Input: part model. Units: mm. Frame: model coordinates. Face numbers are marked on the shaded views. A direction names the side the tool comes from. Round coordinates to 2 decimals unless told otherwise and drop trailing zeros. Order: outer loops, then holes, each group sorted by start corner. A loop starts at its lowest first (then second) coordinate and runs counter-clockwise, first axis right, second up. Notation, with made-up numbers: (-25, 35.25) -> (5, 35.25) arc R5 ccw to (5, 41.25) -> close; hole circle Ø11 at (2.25, 29.5). An arc over 180 degrees is marked (long way). Use a Markdown table: item, result.
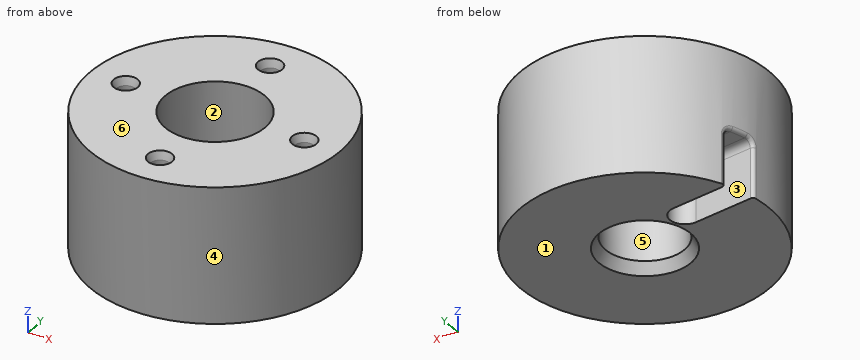
from build123d import *

# Parameters (mm, degrees)
SKETCH_1_R          = 17.5
EXTRUDE_1_DEPTH     = 19
SKETCH_2_R          = 1.3
CUT_EXTRUDE_1_DEPTH = 8
SKETCH_4_R          = 7
CUT_EXTRUDE_3_DEPTH = 9
SKETCH_5_R          = 5.55
CUT_EXTRUDE_4_DEPTH = 10
CUT_EXTRUDE_START   = -8
CUT_EXTRUDE_6_DEPTH = 8
FILLET_1_R          = 1
FILLET_2_R          = 0.5
CHAMFER_1_SIZE      = 0.9
CHAMFER_1_SIZE2     = 1.558845727
CHAMFER_2_SIZE      = 0.4
CHAMFER_2_SIZE2     = 1.098990968


with BuildPart() as part:
    # 草图1 → 凸台-拉伸1 (new body)
    with BuildSketch(Plane.XY):
        Circle(SKETCH_1_R)
    extrude(amount=-EXTRUDE_1_DEPTH)

    # 草图2 → 切除-拉伸1 (cut)
    with BuildSketch(Plane.XY):
        with Locations((12.5, 0)):
            Circle(SKETCH_2_R)
        with Locations((0, -12.5)):
            Circle(SKETCH_2_R)
        with Locations((-12.5, 0)):
            Circle(SKETCH_2_R)
        with Locations((0, 12.5)):
            Circle(SKETCH_2_R)
    extrude(amount=-CUT_EXTRUDE_1_DEPTH, mode=Mode.SUBTRACT)

    # 草图4 → 切除-拉伸3 (cut)
    with BuildSketch(Plane.XY):
        Circle(SKETCH_4_R)
    extrude(amount=-CUT_EXTRUDE_3_DEPTH, mode=Mode.SUBTRACT)

    # 草图5 → 切除-拉伸4 (cut)
    with BuildSketch(Plane.XY.offset(-9)):
        Circle(SKETCH_5_R)
    extrude(amount=-CUT_EXTRUDE_4_DEPTH, mode=Mode.SUBTRACT)

    # 草图11 → 切除-拉伸6 (cut)
    with BuildSketch(Plane(origin=(0, 0, -19), x_dir=(-1, 0, 0), z_dir=(0, 0, -1)).offset(CUT_EXTRUDE_START)):
        with BuildLine():
            ThreePointArc((17.194499347, 3.255640061), (16.671203225, 5.32174624), (15.900621658, 7.308914482))
            Line((15.900621658, 7.308914482), (7.74531425, 6.090095623))
            ThreePointArc((7.74531425, 6.090095623), (5.978780701, 3.702762547), (8.366113777, 1.936228997))
            Line((8.366113777, 1.936228997), (17.194499347, 3.255640061))
        make_face()
    extrude(amount=CUT_EXTRUDE_6_DEPTH, mode=Mode.SUBTRACT)

    # 圆角1
    fillet_1_edges = [part.edges().sort_by_distance(p)[0] for p in [
        (-11.822967954, 6.699505053, -11),
        (-5.978780701, 3.702762547, -11),
        (-12.780306562, 2.595934529, -11),
    ]]
    fillet(fillet_1_edges, radius=FILLET_1_R)

    # 圆角2
    fillet_2_edges = [part.edges().sort_by_distance(p)[0] for p in [
        (-17.194499347, 3.255640061, -15.5),
        (-16.675851852, 5.30716167, -11),
        (-15.900621658, 7.308914482, -15.5),
        (-17.137411019, 3.543888201, -11.292266818),
        (-16.027314009, 7.026749296, -11.28802798),
    ]]
    fillet(fillet_2_edges, radius=FILLET_2_R)

    # 倒角1
    chamfer_1_edges = [part.edges().sort_by_distance(p)[0] for p in [
        (-5.55, 0, -19),
    ]]
    chamfer_1_side = [part.faces().sort_by_distance(p)[0] for p in [
        (-1.349167098, -16.951419764, -19),
    ]]
    chamfer(chamfer_1_edges, length=CHAMFER_1_SIZE, length2=CHAMFER_1_SIZE2, reference=chamfer_1_side[0])

    # 倒角2
    chamfer_2_edges = [part.edges().sort_by_distance(p)[0] for p in [
        (-1.3, -12.5, 0),
        (-13.8, 0, 0),
        (-1.3, 12.5, 0),
        (11.2, 0, 0),
    ]]
    chamfer_2_side = [part.faces().sort_by_distance(p)[0] for p in [
        (-17.005025253, 0, 0),
    ]]
    chamfer(chamfer_2_edges, length=CHAMFER_2_SIZE, length2=CHAMFER_2_SIZE2, reference=chamfer_2_side[0])


solid = part.part
1) Ray query, probe 1 along Y at (x, z) = (0, -2.75); probe 2 along Y at (x, z) = (0, -15); probe 3 along Y at (x, z) = (-0.5, -3.75). Return the intervals inside material, ascending.
Answer key:
| item | result |
|---|---|
| probe 1 | y = -17.5 to -13.8, -11.2 to -7, 7 to 11.2, 13.8 to 17.5 |
| probe 2 | y = -17.5 to -5.55, 5.55 to 17.5 |
| probe 3 | y = -17.49 to -13.7, -11.3 to -6.98, 6.98 to 11.3, 13.7 to 17.49 |
2) Cut plane D-D on x = 12.5. Return loops of the section in (y, z).
Answer key:
| item | result |
|---|---|
| outline | (-12.25, -19) -> (12.25, -19) -> (12.25, 0) -> (1.7, 0) -> (1.3, -1.1) -> (1.3, -8) -> (-1.3, -8) -> (-1.3, -1.1) -> (-1.7, 0) -> (-12.25, 0) -> close |
3) Cut plane C-C on z = -1.75. Return loops of the section in (x, y), and give its area (3 significant figures).
Answer key:
| item | result |
|---|---|
| outline | circle Ø35 at (0, 0); hole circle Ø2.6 at (-12.5, 0); hole circle Ø14 at (0, 0); hole circle Ø2.6 at (0, -12.5); hole circle Ø2.6 at (0, 12.5); hole circle Ø2.6 at (12.5, 0) |
| area | 787 mm^2 |
4) Cut plane A-A on x = 0. Return loops of the section in (y, z), and give its area (3 significant figures).
Answer key:
| item | result |
|---|---|
| outline | (-17.5, -19) -> (-6.45, -19) -> (-5.55, -17.44) -> (-5.55, -9) -> (-7, -9) -> (-7, 0) -> (-10.8, 0) -> (-11.2, -1.1) -> (-11.2, -8) -> (-13.8, -8) -> (-13.8, -1.1) -> (-14.2, 0) -> (-17.5, 0) -> close; (5.55, -17.44) -> (6.45, -19) -> (17.5, -19) -> (17.5, 0) -> (14.2, 0) -> (13.8, -1.1) -> (13.8, -8) -> (11.2, -8) -> (11.2, -1.1) -> (10.8, 0) -> (7, 0) -> (7, -9) -> (5.55, -9) -> close |
| area | 384 mm^2 |
5) Cut plane B-B on z = -16.5. Return loops of the section in (x, y), and give its area (3 significant figures).
Answer key:
| item | result |
|---|---|
| outline | (-17.28, 2.77) arc R17.5 ccw (long way) to (-15.6, 7.93) arc R0.5 ccw to (-15.23, 7.21) -> (-7.75, 6.09) arc R2.1 cw to (-8.37, 1.94) -> (-16.71, 3.18) arc R0.5 ccw to start; hole circle Ø11.1 at (0, 0) |
| area | 822 mm^2 |
6) Draft query along X for the marked faces 4, 5 and 6. Return one class per face: released by +X, released by -X, zero draft, split by the parting line, or undercut.
Answer key:
| item | result |
|---|---|
| face 4 | split by the parting line |
| face 5 | undercut |
| face 6 | zero draft |
7) Set-up query: the marked faces 1, 2 and 3. Return all of +Z, -Z, +X, -X, +Y, -Y with unobstructed straight access to the full face (end or side cutting, diameter ignored); none if empty.
Answer key:
| item | result |
|---|---|
| face 1 | -Z, +X, -X, +Y, -Y |
| face 2 | +Z |
| face 3 | -Z |
8) Contact query for flat-ended pins moving along their axis: P1, Ø8, axis at y = 6.5, z = -5.5, coming from the -X side; P2, Ø10, axis at y = -7, z = -3, coming from the -X side; P3, Ø1.3, axis at x = -0.5, y = -12.5, coming from the +Z side. Output: stop coordinate, or through.
Answer key:
| item | result |
|---|---|
| P1 | stops at x = -17.32 |
| P2 | stops at x = -17.39 |
| P3 | stops at z = -8 |
